Part model, mm, in its own coordinate system. Face numbers are marked on the shaded views. A direction names the side the tool comes from. Round coordinates to 2 decimals unless told otherwise and drop trailing zeros. Write each loop counter-clockwise with the first axis right and the second up, starting at its lowest first coordinate (ties: lowest second). Pieces come first, ordered by that corner, then holes. Notation, with made-up numbers: M -2.75,64 L 18.25,64 A22 cw 18.25,75 Z; hole C 12,37 d11. An arc over 180 degrees is marked long. Answer as a JSON object with one key per item and string values. Group by question number.
1. Drop flat-ended pins along their axis: pin 1 (9 mm diameter, centred on x = -6, z = 14.5, fed in from +Y); pin 2 (5.5 mm diameter, centred on y = 13.47, z = -24.89, fed in from -X); pin 3 (3 mm diameter, centred on x = 0.5, y = 7.5, fed in from +Z). Give the stop position or say it passes through.
2. Drill centre lines: line 1 (X direction, y = -7, z = -33); line 2 (Y direction, x = 5.5, z = -24.89); line 3 (Z direction, x = 3.5, y = 23.47). Where is each one in solid material? Low to high. Write a range as from..to.
3. Band-saw the part on A-A, the plane x = 9. Write the cut outline in (y, z).
4. Which spindle directions (+Z, -Z, +X, -X, +Y, -Y) get a long thin tool onto all of the face, cutting with end or side? Do the marked faces 1, 2 and 3. Say none if no direction does.
5. Two-plate mould, pull along Z, no slides. Class the marked faces 4, 5 and 6: +Z half, -Z half, draft (parallel to the pull), parting line (faces both ways), or undercut.
6. Band-saw the part on C-C, the plane z = -33. Write the cut outline in (x, y).
7. Band-saw the part on D-D, the plane y = -5. Write the cut outline in (x, z).
8. Band-saw the part on B-B, the plane x = -9. Write the cut outline in (y, z), plus the area to 3 significant figures.
from build123d import *

# Parameters (mm, degrees)
SKETCH1_W           = 25
SKETCH1_H           = 60
BOSS_EXTRUDE1_DEPTH = 8
SKETCH2_W           = 25
SKETCH2_H           = 10
SKETCH2_W_2         = 12.5
BOSS_EXTRUDE2_DEPTH = 21
CUT_EXTRUDE1_REACH  = 27
SKETCH3_R           = 1.75
SKETCH6_W           = 30
SKETCH6_H           = 75
BOSS_EXTRUDE3_DEPTH = 10
CUT_EXTRUDE4_REACH  = 12
SKETCH7_R           = 2


with BuildPart() as part:
    # Sketch1 → Boss-Extrude1 (new body)
    with BuildSketch(Plane(origin=(0, 0, 0), x_dir=(1, 0, 0), z_dir=(0, 1, 0))):
        Rectangle(SKETCH1_W, SKETCH1_H)
    extrude(amount=BOSS_EXTRUDE1_DEPTH)

    # Sketch2 → Boss-Extrude2 (add)
    with BuildSketch(Plane(origin=(0, 8, 0), x_dir=(1, 0, 0), z_dir=(0, 1, 0))):
        with Locations((0, -25)):
            Rectangle(SKETCH2_W, SKETCH2_H)
        with Locations((6.25, 25)):
            Rectangle(SKETCH2_W_2, SKETCH2_H)
    extrude(amount=BOSS_EXTRUDE2_DEPTH)

    # Sketch3 → Cut-Extrude1 (cut, up to next)
    with BuildSketch(Plane.ZY.offset(-12.5), mode=Mode.PRIVATE) as cut_extrude1_sk1:
        with Locations((-24.89, 23.47)):
            Circle(SKETCH3_R)
    cut_extrude1_tool1 = extrude(cut_extrude1_sk1.sketch, amount=CUT_EXTRUDE1_REACH, mode=Mode.PRIVATE) & part.part
    add(cut_extrude1_tool1.solids().sort_by_distance((12.5, 23.47, -24.89))[0], mode=Mode.SUBTRACT)
    # Sketch3 → Cut-Extrude1 (cut, up to next)
    with BuildSketch(Plane.ZY.offset(-12.5), mode=Mode.PRIVATE) as cut_extrude1_sk2:
        with Locations((-24.89, 13.47)):
            Circle(SKETCH3_R)
    cut_extrude1_tool2 = extrude(cut_extrude1_sk2.sketch, amount=CUT_EXTRUDE1_REACH, mode=Mode.PRIVATE) & part.part
    add(cut_extrude1_tool2.solids().sort_by_distance((12.5, 13.47, -24.89))[0], mode=Mode.SUBTRACT)
    # Sketch3 → Cut-Extrude1 (cut, up to next)
    with BuildSketch(Plane.ZY.offset(-12.5), mode=Mode.PRIVATE) as cut_extrude1_sk3:
        with Locations((24.89, 23.47)):
            Circle(SKETCH3_R)
    cut_extrude1_tool3 = extrude(cut_extrude1_sk3.sketch, amount=CUT_EXTRUDE1_REACH, mode=Mode.PRIVATE) & part.part
    add(cut_extrude1_tool3.solids().sort_by_distance((12.5, 23.47, 24.89))[0], mode=Mode.SUBTRACT)
    # Sketch3 → Cut-Extrude1 (cut, up to next)
    with BuildSketch(Plane.ZY.offset(-12.5), mode=Mode.PRIVATE) as cut_extrude1_sk4:
        with Locations((24.89, 13.47)):
            Circle(SKETCH3_R)
    cut_extrude1_tool4 = extrude(cut_extrude1_sk4.sketch, amount=CUT_EXTRUDE1_REACH, mode=Mode.PRIVATE) & part.part
    add(cut_extrude1_tool4.solids().sort_by_distance((12.5, 13.47, 24.89))[0], mode=Mode.SUBTRACT)

    # Sketch6 → Boss-Extrude3 (add)
    with BuildSketch(Plane.XZ):
        Rectangle(SKETCH6_W, SKETCH6_H)
    extrude(amount=BOSS_EXTRUDE3_DEPTH)

    # Sketch7 → Cut-Extrude4 (cut, up to next)
    with BuildSketch(Plane(origin=(0, 0, 0), x_dir=(1, 0, 0), z_dir=(0, 1, 0)), mode=Mode.PRIVATE) as cut_extrude4_sk1:
        with Locations((9, 33)):
            Circle(SKETCH7_R)
    cut_extrude4_tool1 = extrude(cut_extrude4_sk1.sketch, amount=-CUT_EXTRUDE4_REACH, mode=Mode.PRIVATE) & part.part
    add(cut_extrude4_tool1.solids().sort_by_distance((9, 0, -33))[0], mode=Mode.SUBTRACT)
    # Sketch7 → Cut-Extrude4 (cut, up to next)
    with BuildSketch(Plane(origin=(0, 0, 0), x_dir=(1, 0, 0), z_dir=(0, 1, 0)), mode=Mode.PRIVATE) as cut_extrude4_sk2:
        with Locations((-9, 33)):
            Circle(SKETCH7_R)
    cut_extrude4_tool2 = extrude(cut_extrude4_sk2.sketch, amount=-CUT_EXTRUDE4_REACH, mode=Mode.PRIVATE) & part.part
    add(cut_extrude4_tool2.solids().sort_by_distance((-9, 0, -33))[0], mode=Mode.SUBTRACT)
    # Sketch7 → Cut-Extrude4 (cut, up to next)
    with BuildSketch(Plane(origin=(0, 0, 0), x_dir=(1, 0, 0), z_dir=(0, 1, 0)), mode=Mode.PRIVATE) as cut_extrude4_sk3:
        with Locations((-9, -33)):
            Circle(SKETCH7_R)
    cut_extrude4_tool3 = extrude(cut_extrude4_sk3.sketch, amount=-CUT_EXTRUDE4_REACH, mode=Mode.PRIVATE) & part.part
    add(cut_extrude4_tool3.solids().sort_by_distance((-9, 0, 33))[0], mode=Mode.SUBTRACT)
    # Sketch7 → Cut-Extrude4 (cut, up to next)
    with BuildSketch(Plane(origin=(0, 0, 0), x_dir=(1, 0, 0), z_dir=(0, 1, 0)), mode=Mode.PRIVATE) as cut_extrude4_sk4:
        with Locations((9, -33)):
            Circle(SKETCH7_R)
    cut_extrude4_tool4 = extrude(cut_extrude4_sk4.sketch, amount=-CUT_EXTRUDE4_REACH, mode=Mode.PRIVATE) & part.part
    add(cut_extrude4_tool4.solids().sort_by_distance((9, 0, 33))[0], mode=Mode.SUBTRACT)


solid = part.part
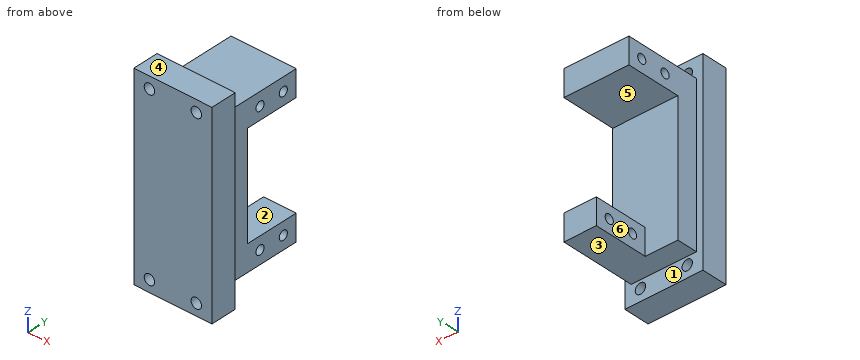
Worked answers:
{
 "1": {"pin 1": "stops at y = 8", "pin 2": "stops at x = 0", "pin 3": "stops at z = 30"},
 "2": {"line 1": "x = -15..-11, -7..7, 11..15", "line 2": "y = -10..11.72, 15.22..21.72, 25.22..29", "line 3": "z = -30..-26.64, -23.14..-20, 20..23.14, 26.64..30"},
 "3": {"outline": "M -10,-37.5 L 0,-37.5 L 0,-35 L -10,-35 Z; M -10,-31 L 0,-31 L 0,-30 L 29,-30 L 29,-20 L 8,-20 L 8,20 L 29,20 L 29,30 L 0,30 L 0,31 L -10,31 Z; M -10,35 L 0,35 L 0,37.5 L -10,37.5 Z; hole C 13.47,-24.89 d3.5; hole C 13.47,24.89 d3.5; hole C 23.47,-24.89 d3.5; hole C 23.47,24.89 d3.5"},
 "4": {"face 1": "+Y", "face 2": "+X, -X, +Y", "face 3": "-Z, +X, -X, +Y"},
 "5": {"face 4": "+Z half", "face 5": "undercut", "face 6": "draft"},
 "6": {"outline": "M -15,-10 L -11,-10 L -11,0 L -15,0 Z; M -7,-10 L 7,-10 L 7,0 L -7,0 Z; M 11,-10 L 15,-10 L 15,0 L 11,0 Z"},
 "7": {"outline": "M -15,-37.5 L 15,-37.5 L 15,37.5 L -15,37.5 Z; hole C -9,-33 d4; hole C -9,33 d4; hole C 9,-33 d4; hole C 9,33 d4"},
 "8": {"outline": "M -10,-37.5 L 0,-37.5 L 0,-35 L -10,-35 Z; M -10,-31 L 0,-31 L 0,-30 L 8,-30 L 8,20 L 29,20 L 29,30 L 0,30 L 0,31 L -10,31 Z; M -10,35 L 0,35 L 0,37.5 L -10,37.5 Z; hole C 13.47,24.89 d3.5; hole C 23.47,24.89 d3.5", "area": "1,340 mm^2"}
}
